Check sheet for the modelled part. Datum: model origin and axes. Units: mm. A direction names the side the tool comes from. Give positions to 0.01 mm unless a question says otherwise; leave off trailing zeros. Loops run counter-clockwise (first coordinate to the right, second up) from the corner with the lowest first, then second, coordinate; pieces in that order, holes last. Notation, with made-up numbers: (18.25, 73) -> (32.25, 73) arc R18 cw to (32.25, 101) -> close; hole circle Ø9 at (4, 12.25). An arc over 180 degrees is marked (long way). Answer as CSV lines item,"result". Start each with the question number.
(1) Section check B-B on x = 0. Enter the section's corners in (y, z).
(2) Gauge pin test, flat ends, axial feed: pin 1 Ø2 at (y, z) = (-12.5, -3) entering from -X; pin 2 Ø3 at (y, z) = (-33.5, 7) entering from +X; pin 3 Ø6.5 at (x, z) = (0.5, 5) entering from +Y; pin 4 Ø1 at (x, z) = (-3.5, 1.5) entering from +Y. Record the tip position at first contact, or that the pin passes through.
(3) Section check D-D on x = -7. Enter the section's corners in (y, z), plus the area to 3 significant figures.
(4) Section check A-A on z = 0. Enter the section's corners in (x, y).
(5) Section check C-C on y = -1. Enter the section's corners in (x, z).
(6) Material ranges on line 1 (Y direction, x = -8.5, z = 5.75); line 2 (X direction, y = -38.5, z = 0); line 3 (Z direction, x = 3.75, y = -13.5), recorded low to high. Write a range as from..to.
(7) Access from +Z, -Z, +X, -X, +Y, -Y to the whole of each face (thin tool, end or side, straight path). Record for faces 1 (the face through (9.274, -41.192, 2.059)), 2 (the face through (5, 12, 5)).
(8) Release check for a two-part mould opening along Y. For faces 3 (the face through (9, -41.75, 5)), 4 (the face through (5, -45, 5)), 5 (the face through (-3.2, 10.4, -10)), 6 (the face through (9.274, 8.192, 2.059)) record: pulls with the +Y half, pulls with the -Y half, needs draft (parallel to the pull), parting line crosses it, or undercut.
from build123d import *


with BuildPart() as part:
    # Sketch1 → Revolve1 (revolve)
    with BuildSketch(Plane.XY, mode=Mode.PRIVATE) as revolve1_sk:
        Polygon((6, -16.5), (6, 12), (10.5, 12), (10.5, 8.75), (9.5, 8.75), (9.5, 7.65), (10.5, 7.65), (10.5, -16.5), align=None)
    revolve1 = revolve(revolve1_sk.sketch.rotate(Axis((0, 0, 0), (0, 1, 0)), 90), axis=Axis((0, 0, 0), (0, 1, 0)))

    # Mirror1: Revolve1 across plane
    add(revolve1.mirror(Plane(origin=(6, -16.5, 0), x_dir=(0, 0, 1), z_dir=(0, -1, 0))))


solid = part.part
Working result:
1,outline,"(-45, -10.5) -> (-41.75, -10.5) -> (-41.75, -9.5) -> (-40.65, -9.5) -> (-40.65, -10.5) -> (7.65, -10.5) -> (7.65, -9.5) -> (8.75, -9.5) -> (8.75, -10.5) -> (12, -10.5) -> (12, -6) -> (-45, -6) -> close; (-45, 6) -> (12, 6) -> (12, 10.5) -> (8.75, 10.5) -> (8.75, 9.5) -> (7.65, 9.5) -> (7.65, 10.5) -> (-40.65, 10.5) -> (-40.65, 9.5) -> (-41.75, 9.5) -> (-41.75, 10.5) -> (-45, 10.5) -> close"
2,pin 1,"stops at x = -10.31"
2,pin 2,"stops at x = 8.94"
2,pin 3,"stops at y = 12"
2,pin 4,"passes through"
3,outline,"(-45, -7.83) -> (-41.75, -7.83) -> (-41.75, -6.42) -> (-40.65, -6.42) -> (-40.65, -7.83) -> (7.65, -7.83) -> (7.65, -6.42) -> (8.75, -6.42) -> (8.75, -7.83) -> (12, -7.83) -> (12, 7.83) -> (8.75, 7.83) -> (8.75, 6.42) -> (7.65, 6.42) -> (7.65, 7.83) -> (-40.65, 7.83) -> (-40.65, 6.42) -> (-41.75, 6.42) -> (-41.75, 7.83) -> (-45, 7.83) -> close"
3,area,"886 mm^2"
4,outline,"(-10.5, -45) -> (-6, -45) -> (-6, 12) -> (-10.5, 12) -> (-10.5, 8.75) -> (-9.5, 8.75) -> (-9.5, 7.65) -> (-10.5, 7.65) -> (-10.5, -40.65) -> (-9.5, -40.65) -> (-9.5, -41.75) -> (-10.5, -41.75) -> close; (6, -45) -> (10.5, -45) -> (10.5, -41.75) -> (9.5, -41.75) -> (9.5, -40.65) -> (10.5, -40.65) -> (10.5, 7.65) -> (9.5, 7.65) -> (9.5, 8.75) -> (10.5, 8.75) -> (10.5, 12) -> (6, 12) -> close"
5,outline,"circle Ø21 at (0, 0); hole circle Ø12 at (0, 0)"
6,line 1,"y = -45..-41.75, -40.65..7.65, 8.75..12"
6,line 2,"x = -10.5..-6, 6..10.5"
6,line 3,"z = -9.81..-4.68, 4.68..9.81"
7,face 1,"none"
7,face 2,"+Z, -Z, +X, -X, +Y"
8,face 3,"undercut"
8,face 4,"pulls with the -Y half"
8,face 5,"needs draft"
8,face 6,"undercut"
